For this review, take the finished solid that the model builds, in its own axes (mm). A direction names the side the tool comes from. Coordinates: 2 decimals unless noted, no trailing zeros. Order: outer loops, then holes, each group sorted by start corner. A loop starts at its lowest first (then second) coordinate and runs counter-clockwise, first axis right, second up. Notation, with made-up numbers: (-29, -24) - (-18, -24) arc R23 ccw to (-18, -13) - close; hole circle Ø2 at (-25.5, 72.25). An arc over 180 degrees is marked (long way). One line per item, written item: value. Start each with the question number.
(1) Mouldability with a two-part tool opening along Y and no side actions: class faces 4 (the flat face through (-142.43, -10.26, 0.02)), 5 (the flat face through (-109.325, -50.508, 0.022)), 6 (the cylindrical face through (-44.743, -85.812, 0.022)) as released by +Y, released by -Y, zero draft, split by the parting line, or undercut.
(2) Clearance check with flat-ended pins moving along their axes: pin 1 (1 mm diameter, centred on y = -3, z = -0.5, fed in from +X); pin 2 (1 mm diameter, centred on y = -107.5, z = 1, fed in from +X); pin 3 (1 mm diameter, centred on x = -93, z = 0.5, fed in from -Y). State where each tip first meets the part, or that it passes through.
(3) Consider section A-A on x = -22.5. Write out the cut boundary in (y, z), then the cut area to 3 significant figures.
(4) To check wall thickness, follow line 1 along Y through (x, z) = (-40, -0.15); line 2 along X through (y, z) = (25, 0.25); line 3 along Y through (x, z) = (-26, -0.9). State the ranges of each line that lie inside material, in increasing order.
(5) For faces 1 (the flat face through (-122, 24, 1.588)), 2 (the flat face through (-110.85, -40.29, -0.02)), 3 (the flat face through (-96.81, -36.1, 0.02)), list the 3-axis set-ups (+Z, -Z, +X, -X, +Y, -Y) from which the entire face can be reached by the end or side of a thin tool; tool diameter is ignored.
(6) Consider section C-C on x = -63. Write out the cut boundary in (y, z), then the cut area to 3 significant figures.
(7) Consider section D-D on y = -69. Write out the cut boundary in (x, z), then the cut area to 3 significant figures.
```python
from build123d import *

# Parameters (mm, degrees)
BOSS_EXTRUDE1_DEPTH = 1.5875
CUT_EXTRUDE1_DEPTH  = 3.175
FILLET1_R           = 8.89
SKETCH3_W           = 234.443386257
SKETCH3_H           = 422.563019086
CUT_EXTRUDE2_DEPTH  = 206.876411182
BOSS_EXTRUDE2_DEPTH = 1.5875
FILLET2_R           = 6.35
FILLET3_R           = 12.7
SKETCH6_W           = 3.302
SKETCH6_H           = 12.7
CUT_EXTRUDE3_DEPTH  = 215.861709895


with BuildPart() as part:
    # Sketch1 → Boss-Extrude1 (new, symmetric)
    with BuildSketch(Plane.XY):
        with BuildLine():
            Line((-120.187952283, -34.272453), (-99.98237601, -54.478029272))
            Line((-99.98237601, -54.478029272), (-101.142590553, -63.40953887))
            ThreePointArc((-101.142590553, -63.40953887), (-81.179103762, -82.298079227), (-57.767453, -96.692952283))
            ThreePointArc((-57.767453, -96.692952283), (94.292689271, 117.787689271), (-120.187952283, -34.272453))
        make_face()
    extrude(amount=BOSS_EXTRUDE1_DEPTH, both=True)

    # Sketch2 → Cut-Extrude1 (cut)
    with BuildSketch(Plane.XY.offset(1.5875)):
        with BuildLine():
            Line((-83.903310386, -49.004480206), (-85.12178765, -58.384505172))
            ThreePointArc((-85.12178765, -58.384505172), (97.723123527, 89.828726174), (-107.51910025, -25.388690342))
            Line((-107.51910025, -25.388690342), (-83.903310386, -49.004480206))
        make_face()
    extrude(amount=-CUT_EXTRUDE1_DEPTH, mode=Mode.SUBTRACT)

    # Fillet1
    fillet1_edges = [part.edges().sort_by_distance(p)[0] for p in [
        (-83.903310386, -49.004480206, 0),
        (-107.51910025, -25.388690342, 0),
        (-85.12178765, -58.384505172, 0),
        (-99.98237601, -54.478029272, -0.79375),
        (-120.187952283, -34.272453, -0.79375),
        (-101.142590553, -63.40953887, -0.79375),
    ]]
    fillet(fillet1_edges, radius=FILLET1_R)

    # Sketch3 → Cut-Extrude2 (cut, through all)
    with BuildSketch(Plane(origin=(0, 0, 0), x_dir=(0, 0, -1), z_dir=(1, 0, 0))):
        with Locations((10.168628802, 16.433452221)):
            Rectangle(SKETCH3_W, SKETCH3_H)
    extrude(amount=CUT_EXTRUDE2_DEPTH, mode=Mode.SUBTRACT)

    # Sketch5 → Boss-Extrude2 (add, symmetric)
    with BuildSketch(Plane.XY):
        Polygon((-146.81661939, -13.003405573), (-125.293457687, 0.445758531), (-91.969146245, -50.60762416), (-100.600425128, -59.235866221), align=None)
    extrude(amount=BOSS_EXTRUDE2_DEPTH, both=True)

    # Fillet2
    # the kernel refuses this fillet: 6.35 mm, written as the material it adds along each edge
    with BuildSketch(Plane(origin=(-100.600425128, -59.235866221, -1.5875), x_dir=(-0.03079411224323655, -0.9995257488685076, 0), z_dir=(0, 0, 1)), Plane(origin=(-100.600425128, -59.235866221, 0), x_dir=(-0.03079411224323655, -0.9995257488685076, 0), z_dir=(0, 0, 1))) as fillet2_piece_1:
        with BuildLine():
            CenterArc((2.784435169, -6.30796831), FILLET2_R, 96.595975588, 40.158594829)
            Line((-1.841067542, -1.957425279), (-2.303617813, -1.522370976))
            Line((-2.303617813, -1.522370976), (-0.462550271, 0.435054303))
            Line((-0.462550271, 0.435054303), (0.062369909, 0.63192958))
            ThreePointArc((0.062369909, 0.63192958), (0.223047541, 0.61607109), (1.982086545, 0.630796831))
            Line((1.982086545, 0.630796831), (2.055027329, 0))
        make_face()
    extrude(amount=1.5875)

    # Fillet3
    fillet3_edges = [part.edges().sort_by_distance(p)[0] for p in [
        (-130.70446004, -2.935411002, 0),
    ]]
    fillet(fillet3_edges, radius=FILLET3_R)

    # Sketch6 → Cut-Extrude3 (cut, through all)
    with BuildSketch(Plane(origin=(0, 0, -1.5875), x_dir=(-1, 0, 0), z_dir=(0, 0, -1))):
        with Locations((1.651, 154.305)):
            Rectangle(SKETCH6_W, SKETCH6_H)
        Polygon((105.489605782, 89.621888205), (107.18979641, 86.702712453), (118.164141341, 93.094406542), (116.463950713, 96.013582294), align=None)
        Polygon((105.201667309, -36.998635355), (106.90185793, -34.079459599), (128.850547824, -46.862847722), (127.150357204, -49.782023478), align=None)
        with Locations((1.651, -107.315)):
            Rectangle(SKETCH6_W, SKETCH6_H)
    extrude(amount=-CUT_EXTRUDE3_DEPTH, mode=Mode.SUBTRACT)


solid = part.part
```
Geometry check:
1. face 4: released by +Y
1. face 5: released by -Y
1. face 6: undercut
2. pin 1: stops at x = -114.98
2. pin 2: stops at x = -3.3
2. pin 3: stops at y = -72.56
3. outline: (-107.94, -1.59) - (-92.45, -1.59) - (-92.45, 1.59) - (-107.94, 1.59) - close; (139.44, -1.59) - (154.93, -1.59) - (154.93, 1.59) - (139.44, 1.59) - close
3. area: 98.4 mm^2
4. line 1: y = -103.71 to -87.64, 134.63 to 150.7
4. line 2: x = -133.34 to -118.1
4. line 3: y = -107.3 to -91.72, 138.71 to 154.29
5. face 1: +Z, +X, -X, +Y, -Y
5. face 2: +Z, -Z
5. face 3: +Z, -Z, +X
6. outline: (-94.03, -1.59) - (-76.41, -1.59) - (-76.41, 1.59) - (-94.03, 1.59) - close; (123.4, -1.59) - (141.02, -1.59) - (141.02, 1.59) - (123.4, 1.59) - close
6. area: 112 mm^2
7. outline: (-96.06, -1.59) - (-73.45, -1.59) - (-73.45, 1.59) - (-96.06, 1.59) - close
7. area: 71.8 mm^2
